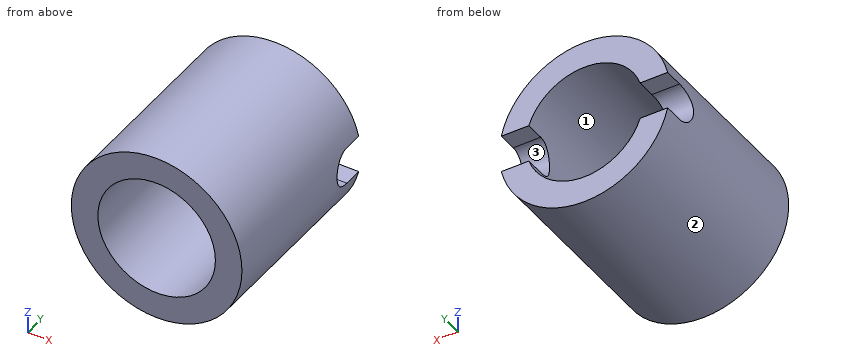
from build123d import *
from build123d.topology import SkipClean

# Parameters (mm, degrees)
SKETCH_1_R               = 4.5
SKETCH_1_R_2             = 3
EXTRUDE_1_DEPTH          = 9
CUT_EXTRUDE_3_DEPTH      = 12.022703843
CUT_EXTRUDE_3_DEPTH_BACK = 12.022703843
SKETCH_2_R               = 1
EXTRUDE_2_DEPTH          = 1
MOVE_FACE_1_OUTLINE_R    = 3.1
MOVE_FACE_1_OUTLINE_R_2  = 3
MOVE_FACE_1_DEPTH        = 10


# Read off the part's stored shape, not the designer's step: 面の移動1
with BuildPart() as part:
    # ｽｹｯﾁ1 → ﾎﾞｽ - 押し出し1 (new body)
    with BuildSketch(Plane(origin=(0, 0, 0), x_dir=(1, 0, 0), z_dir=(0, 1, 0))):
        with Locations(Location((0, 0, 0), (0, 0, 270))):
            Circle(SKETCH_1_R)
        with Locations(Location((0, 0, 0), (0, 0, 270))):
            Circle(SKETCH_1_R_2, mode=Mode.SUBTRACT)
    extrude(amount=EXTRUDE_1_DEPTH)

    # ｽｹｯﾁ2 → ｶｯﾄ - 押し出し3 (cut, two sides: drawn at the far end of the back side and taken through both)
    with BuildSketch(Plane(origin=(0, 0, 0), x_dir=(0, 0, -1), z_dir=(1, 0, 0)).offset(-CUT_EXTRUDE_3_DEPTH_BACK)):
        with Locations((0, 9)):
            Circle(SKETCH_2_R)
    extrude(amount=CUT_EXTRUDE_3_DEPTH + CUT_EXTRUDE_3_DEPTH_BACK, mode=Mode.SUBTRACT)

    # ｽｹｯﾁ3 → ﾎﾞｽ - 押し出し2 (add)
    with SkipClean():  # the faces are left unmerged after this step: merging them gives an invalid solid
        with BuildSketch(Plane(origin=(0, 9, 0), x_dir=(1, 0, 0), z_dir=(0, 1, 0))):
            with BuildLine():
                Line((-2.828427125, -1), (-4.387482194, -1))
                ThreePointArc((-4.387482194, -1), (0, -4.5), (4.387482194, -1))
                Line((4.387482194, -1), (2.828427125, -1))
                ThreePointArc((2.828427125, -1), (0, -3), (-2.828427125, -1))
            make_face()
            with BuildLine():
                Line((2.828427125, 1), (4.387482194, 1))
                ThreePointArc((4.387482194, 1), (0, 4.5), (-4.387482194, 1))
                Line((-4.387482194, 1), (-2.828427125, 1))
                ThreePointArc((-2.828427125, 1), (0, 3), (2.828427125, 1))
            make_face()
        extrude(amount=EXTRUDE_2_DEPTH)

    # Move Face 1 outline → Move Face 1 (cut)
    with BuildSketch(Plane(origin=(0, 0, 0), x_dir=(1, 0, 0), z_dir=(0, 1, 0))):
        Circle(MOVE_FACE_1_OUTLINE_R)
        Circle(MOVE_FACE_1_OUTLINE_R_2, mode=Mode.SUBTRACT)
    extrude(amount=MOVE_FACE_1_DEPTH, mode=Mode.SUBTRACT)


solid = part.part
Design review of the part built by this model. Coordinates are the model's own, in mm. Face numbers are marked on the shaded views. Round coordinates to 2 decimals unless told otherwise and drop trailing zeros. Write each loop counter-clockwise with the first axis right and the second up, starting at its lowest first coordinate (ties: lowest second). Pieces come first, ordered by that corner, then holes. Notation, with made-up numbers: (28, 28.5) -> (41, 28.5) arc R18 ccw to (41, 41.5) -> close; hole circle Ø5 at (77, 24.5). An arc over 180 degrees is marked (long way). One line per item, written item: value. Start each with the question number.
Q1. Add section D-D (x = 3.5). Give the boundary of the cut face in (y, z), then the cut area to 3 significant figures.
Q2. To check wall thickness, follow probe 1 along X at (y, z) = (4.75, -1); probe 2 along X at (y, z) = (2.5, 0). State the ranges of each line that lie inside material, in increasing order.
Q3. The part is to be moulded in two halves that separate along X. For the marked faces 1, 2 and 3, say which applies: pulls with the +X half, pulls with the -X half, needs draft (parallel to the pull), parting line crosses it, or undercut.
Q4. Add section B-B (z = 0). Give the boundary of the cut face in (x, y), then the cut area to 3 significant figures.
Q5. Add section A-A (x = 0). Give the boundary of the cut face in (y, z).
Q6. Add section C-C (y = 7.25). Give the boundary of the cut face in (x, z).
Q7. Insertion check: P1, Ø0.8, axis at x = -3.5, y = 9.5, coming from the +Z side; P2, Ø4, axis at x = 0, z = -3, coming from the +Y side; P3, Ø1.1, axis at x = -4, y = 9.5, coming from the -Z side. Each pin has a flat end and moves straight along its axis. Give the tip position at first contact, or say it passes through.
Response:
1. outline: (0, -2.83) -> (10, -2.83) -> (10, -1) -> (9, -1) arc R1 cw to (9, 1) -> (10, 1) -> (10, 2.83) -> (0, 2.83) -> close
1. area: 53.0 mm^2
2. probe 1: x = -4.39 to -2.93, 2.93 to 4.39
2. probe 2: x = -4.5 to -3.1, 3.1 to 4.5
3. face 1: undercut
3. face 2: parting line crosses it
3. face 3: needs draft
4. outline: (-4.5, 0) -> (-3.1, 0) -> (-3.1, 8) -> (-4.5, 8) -> close; (3.1, 0) -> (4.5, 0) -> (4.5, 8) -> (3.1, 8) -> close
4. area: 22.4 mm^2
5. outline: (0, -4.5) -> (10, -4.5) -> (10, -3.1) -> (0, -3.1) -> close; (0, 3.1) -> (10, 3.1) -> (10, 4.5) -> (0, 4.5) -> close
6. outline: circle Ø9 at (0, 0); hole circle Ø6.2 at (0, 0)
7. P1: stops at z = 3.26
7. P2: stops at y = 10
7. P3: stops at z = -2.89
